For this review, use the dimensioned drawing (mm, ordinates from the lowest corner) and the shaded views. A direction names the side the tool comes from. Coordinates: 2 decimals unless noted, no trailing zeros. Write each loop counter-clockwise with the first axis right and the second up, starting at its lowest first coordinate (ties: lowest second). Pieces come first, ordered by that corner, then holes. Notation, with made-up numbers: M 22.5,18.5 L 59.5,18.5 A12 ccw 59.5,25.5 Z; hole C 63,54.25 d10. An arc over 180 degrees is marked long. One line per question, with ' | ' between items.
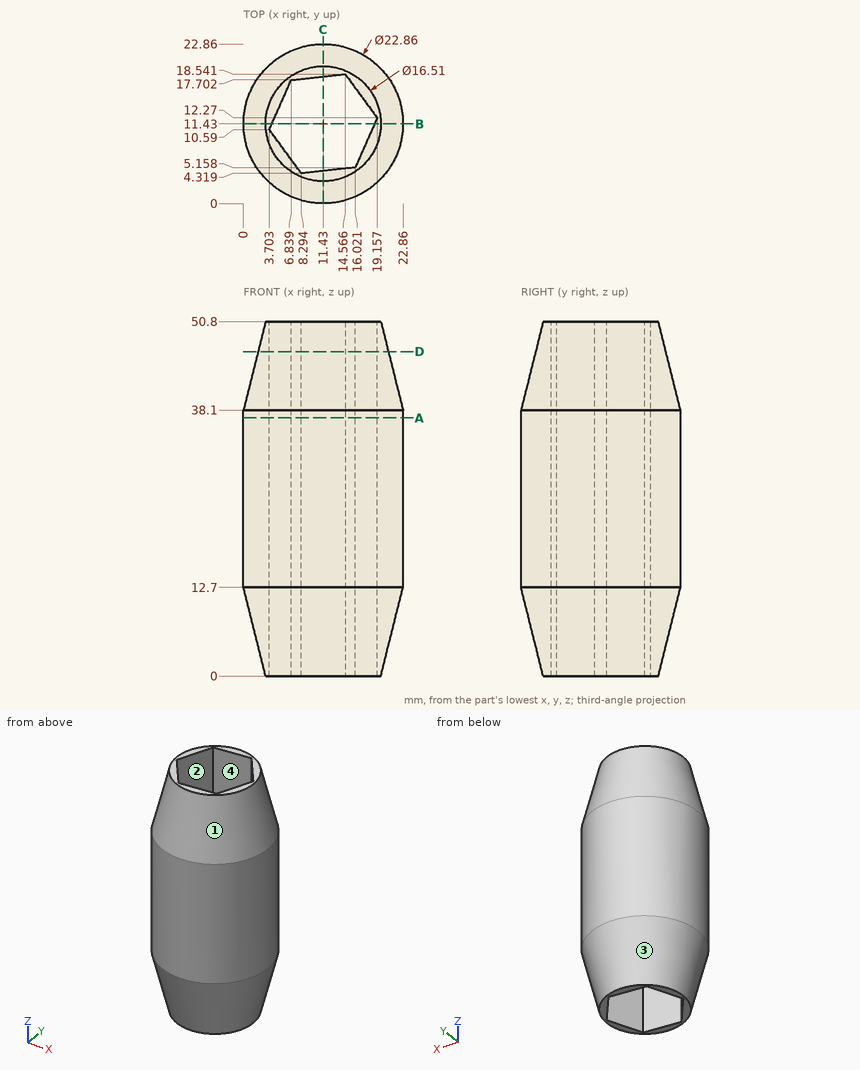
1. Take a section at C-C (x = 11.43). Write out the cut boundary in (y, z) (1 decimal).
Answer sheet:
outline: M 0,12.7 L 3.2,0 L 4.7,0 L 4.7,50.8 L 3.2,50.8 L 0,38.1 Z; M 18.2,0 L 19.7,0 L 22.9,12.7 L 22.9,38.1 L 19.7,50.8 L 18.2,50.8 Z
2. Take a section at A-A (z = 37). Write out the cut boundary in (x, y).
Answer sheet:
outline: C 11.43,11.43 d22.86; hole M 3.7,10.59 L 8.29,4.32 L 16.02,5.16 L 19.16,12.27 L 14.57,18.54 L 6.84,17.7 Z
3. Take a section at B-B (y = 11.43). Write out the cut boundary in (x, z) (1 decimal).
Answer sheet:
outline: M 0,12.7 L 3.2,0 L 4.1,0 L 4.1,50.8 L 3.2,50.8 L 0,38.1 Z; M 18.8,0 L 19.7,0 L 22.9,12.7 L 22.9,38.1 L 19.7,50.8 L 18.8,50.8 Z
4. Draft analysis for pull direction Y (two halves, no side actions). For the marked faces 1 and 2, state which applies: pulls with the +Y half, pulls with the -Y half, needs draft (parallel to the pull), parting line crosses it, or undercut.
Answer sheet:
face 1: parting line crosses it | face 2: undercut
5. To check wall thickness, follow line 1 along X through (y, z) = (9.75, 24) (1 decimal); line 2 along X through (y, z) = (7, 32) (1 decimal); line 3 along Y through (x, z) = (4, 35) (1 decimal). State the ranges of each line that lie inside material, in increasing order. Write a range as [from, to].
Answer sheet:
line 1: [0.1, 4.3], [18, 22.7] | line 2: [0.9, 6.3], [16.8, 22] | line 3: [2.7, 10.2], [11.3, 20.1]
6. Tool access review of the marked faces 3 and 4: name each direction out of +Z, -Z, +X, -X, +Y, -Y from which nothing blocks a thin tool from reaching the whole face with its end or side.
Answer sheet:
face 3: -Z | face 4: +Z, -Z
7. Insertion check: pin 1 Ø10 at (x, z) = (4.5, 11) entering from -Y; pin 2 Ø6 at (y, z) = (5, 16.5) entering from +X; pin 3 Ø12 at (x, z) = (7.5, 43.5) entering from +Y (1 decimal). Each pin has a flat end and moves straight along its axis. Give the tip position at first contact, or say it passes through.
Answer sheet:
pin 1: y = 0.22 | pin 2: x = 22.33 | pin 3: y = 22.8
8. Take a section at D-D (z = 46.5). Write out the cut boundary in (x, y).
Answer sheet:
outline: C 11.43,11.43 d18.66; hole M 3.7,10.59 L 8.29,4.32 L 16.02,5.16 L 19.16,12.27 L 14.57,18.54 L 6.84,17.7 Z
